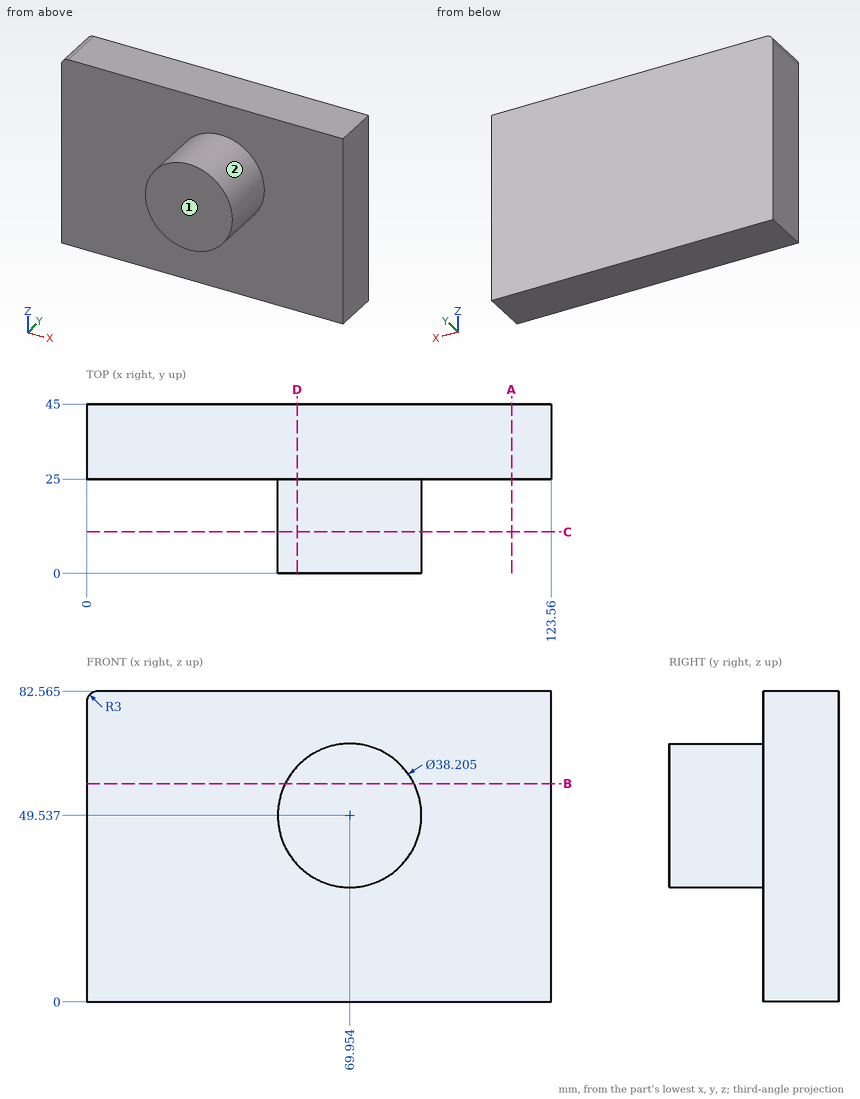
Geometry check sheet. Reference: drawing and pictorial views, mm from the part's lowest x, y, z. A direction names the side the tool comes from. Round coordinates to 2 decimals unless told otherwise and drop trailing zeros. Loops run counter-clockwise (first coordinate to the right, second up) from the corner with the lowest first, then second, coordinate; pieces in that order, holes last. Notation, with made-up numbers: (-36, 86.25) - (16, 86.25) arc R20 ccw to (16, 100.25) - close; hole circle Ø1 at (77.5, 13). An arc over 180 degrees is marked (long way). Use a Markdown table: item, result. Add a question column.
1. Section check D-D, the plane x = 56. Record the boundary of the cut face in (y, z) (1 decimal), plus the area to 3 significant figures.
2. Section check C-C, the plane y = 11. Record the boundary of the cut face in (x, z) (1 decimal), plus the area to 3 significant figures.
3. Access from +Z, -Z, +X, -X, +Y, -Y to the whole of each face (thin tool, end or side, straight path). Record for the marked faces 1 and 2.
4. Section check A-A, the plane x = 113. Record the boundary of the cut face in (y, z) (1 decimal).
5. Gauge pin test, flat ends, axial feed: pin 1 (5 mm diameter, centred on x = 51, y = 7, fed in from -Z) (1 decimal); pin 2 (1 mm diameter, centred on x = 31.5, z = 60.5, fed in from -Y). Record the tip position at first contact, or that the pin passes through.
6. Thickness scan on probe 1 along Y at (x, z) = (20.5, 28); probe 2 along Z at (x, y) = (87, 11.5) (1 decimal); probe 3 along X at (y, z) = (24.5, 43.5). Record the ranges inside material, lowest first. Write a range as [from, to].
7. Section check B-B, the plane z = 58. Record the boundary of the cut face in (x, y), plus the area to 3 significant figures.
Checks:
| question | item | result |
|---|---|---|
| 1 | outline | (0, 36.5) - (25, 36.5) - (25, 0) - (45, 0) - (45, 82.6) - (25, 82.6) - (25, 62.6) - (0, 62.6) - close |
| 1 | area | 2,300 mm^2 |
| 2 | outline | circle Ø38.2 at (70, 49.5) |
| 2 | area | 1,150 mm^2 |
| 3 | face 1 | +Z, -Z, +X, -X, -Y |
| 3 | face 2 | -Y |
| 4 | outline | (25, 0) - (45, 0) - (45, 82.6) - (25, 82.6) - close |
| 5 | pin 1 | stops at z = 39.8 |
| 5 | pin 2 | stops at y = 25 |
| 6 | probe 1 | y = [25, 45] |
| 6 | probe 2 | z = [40.9, 58.2] |
| 6 | probe 3 | x = [51.83, 88.08] |
| 7 | outline | (0, 25) - (52.83, 25) - (52.83, 0) - (87.08, 0) - (87.08, 25) - (123.56, 25) - (123.56, 45) - (0, 45) - close |
| 7 | area | 3,330 mm^2 |
